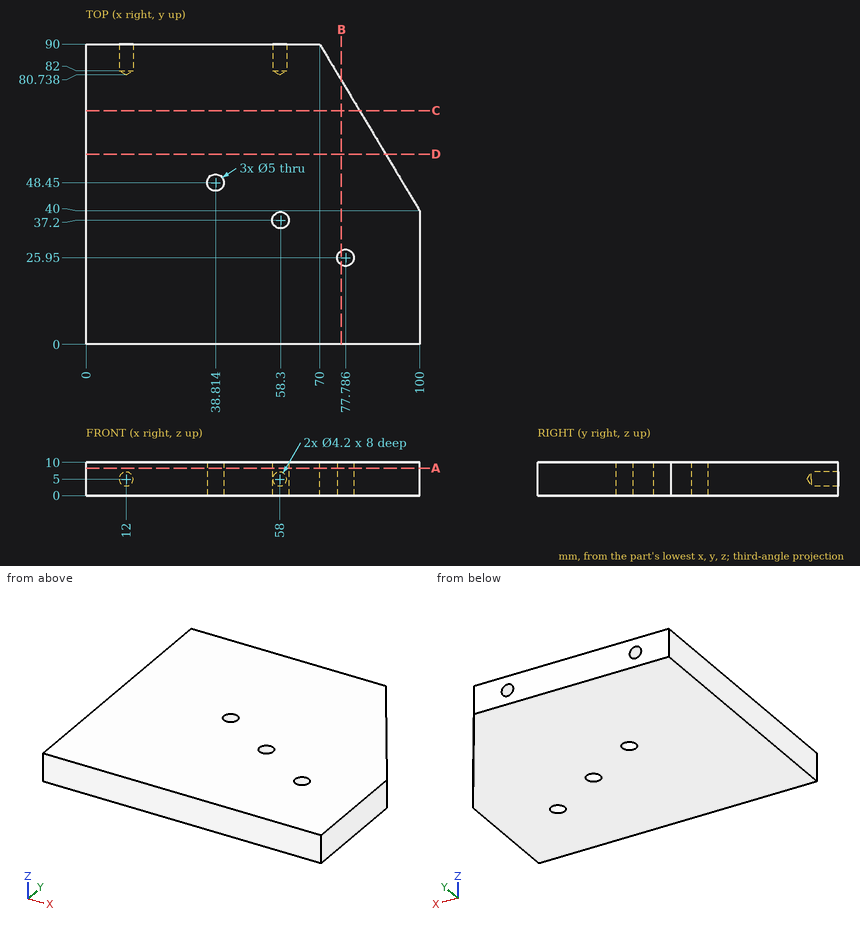
Study the drawing (mm; zero at the part's minimum x, y, z) and answer. Give positions to 0.01 mm unless a question says otherwise; leave off trailing zeros. Loops run counter-clockwise (first coordinate to the right, second up) from the corner with the lowest first, then second, coordinate; pieces in that order, holes last. Notation, with made-up numbers: (-39, 37.5) - (-30, 37.5) arc R12 cw to (-30, 59.5) - close; hole circle Ø9 at (-20.5, 60). An arc over 180 degrees is marked (long way). Answer in a Markdown table with one row per item. Add a question column.
Q1. The part is cut by section D-D (y = 57). Determine the outline of the cut face in (x, z), and give its area (3 significant figures).
Q2. The part is cut by section B-B (x = 76.5). Determine the outline of the cut face in (y, z).
Q3. Each of these flat-tipped pins is pushed along its axis until it touches: P1, Ø5, axis at x = 89, z = 8.5, coming from the +Y side; P2, Ø1.5, axis at y = 33, z = 1, coming from the -X side; P3, Ø4, axis at x = 12, z = 5, coming from the +Y side; P4, Ø3, axis at y = 75, z = 4.5, coming from the +X side. Where does it stop, or does it pass through?
Q4. The part is cut by section A-A (z = 8.25). State how many separate pieces and enclosed holes the cut face has, and give its area (3 significant figures).
Q5. Consider line 1 along Z through (x, y) = (12, 84.5); line 2 along Z through (x, y) = (59, 84.5) (1 decimal); line 3 along Y through (x, z) = (58.3, 5.25). Determine where each line is inside the solid, lowest interval first.
Q6. The part is cut by section C-C (y = 70). Determine the outline of the cut face in (x, z), and give its area (3 significant figures).
Solution:
| question | item | result |
|---|---|---|
| 1 | outline | (0, 0) - (89.8, 0) - (89.8, 10) - (0, 10) - close |
| 1 | area | 898 mm² |
| 2 | outline | (0, 0) - (23.81, 0) - (23.81, 10) - (0, 10) - close; (28.09, 0) - (79.17, 0) - (79.17, 10) - (28.09, 10) - close |
| 3 | P1 | stops at y = 62.5 |
| 3 | P2 | stops at x = 0 |
| 3 | P3 | stops at y = 81.94 |
| 3 | P4 | stops at x = 79.9 |
| 4 | separate pieces | 1 |
| 4 | enclosed holes | 3 |
| 4 | area | 8,190 mm² |
| 5 | line 1 | z = 0 to 2.9, 7.1 to 10 |
| 5 | line 2 | z = 0 to 3.2, 6.8 to 10 |
| 5 | line 3 | y = 0 to 34.7, 39.7 to 80.97 |
| 6 | outline | (0, 0) - (82, 0) - (82, 10) - (0, 10) - close |
| 6 | area | 820 mm² |
